from build123d import *

# Parameters (mm, degrees)
SKETCH_1_R                   = 12.5
EXTRUDE_1_DEPTH              = 20
HOLE_WIZARD_M2_1_D           = 2.4
HOLE_WIZARD_M2_1_CBORE_D     = 6
HOLE_WIZARD_M2_1_CBORE_DEPTH = 0.5


with BuildPart() as part:
    # 草图1 → 凸台-拉伸1 (new body)
    with BuildSketch(Plane.XY):
        Polygon((-340.66541114, -145.626712598), (-330.66541114, -145.626712598), (-330.66541114, -165), (-290.66541114, -165), (-290.66541114, -145.626712598), (-280.66541114, -145.626712598), (-280.66541114, -130), (-340.66541114, -130), align=None)
        with Locations((-310.66541114, -150)):
            Circle(SKETCH_1_R, mode=Mode.SUBTRACT)
    extrude(amount=EXTRUDE_1_DEPTH)

    # M2 六角头螺栓的柱形沉头孔1 (through all)
    with Locations(Plane(origin=(0, -145.626712598, 0), x_dir=(-1, 0, 0), z_dir=(0, -1, 0))):
        with Locations((335.897321014, -10), (285.620390856, -10)):
            CounterBoreHole(HOLE_WIZARD_M2_1_D / 2, HOLE_WIZARD_M2_1_CBORE_D / 2, HOLE_WIZARD_M2_1_CBORE_DEPTH)


solid = part.part
For this review, take the finished solid that the model builds, in its own axes (mm). A direction names the side the tool comes from. Give positions to 0.01 mm unless a question says otherwise; leave off trailing zeros. Loops run counter-clockwise (first coordinate to the right, second up) from the corner with the lowest first, then second, coordinate; pieces in that order, holes last. Notation, with made-up numbers: M 34,75.25 L 51,75.25 A28 cw 51,109.25 Z; hole C -31,-1 d10. An arc over 180 degrees is marked long. Answer as a JSON object with one key per item and string values. Group by question number.
Q1. Mouldability with a two-part tool opening along X and no side actions: class faces 1 (the flat face through (-280.665, -138, 10)), 2 (the flat face through (-311, -136, 20)), 3 (the flat face through (-337, -145.127, 11)), 4 (the flat face through (-287, -145.127, 10)) as +X half, -X half, draft (parallel to the pull), parting line (faces both ways), or undercut.
Q2. Add section A-A on z = 10. Give the boundary of the cut face in (x, y).
Q3. Add section C-C on z = 1.5. Give the boundary of the cut face in (x, y).
Q4. Add section B-B on y = -150. Give the boundary of the cut face in (x, z).
Q5. Tool access review of faces 5 (the flat face through (-333.5, -145.627, 7.6)), 6 (the cylindrical face through (-282.623, -145.38, 9.868)), 7 (the flat face through (-288, -145.627, 7.6)): name each direction out of +Z, -Z, +X, -X, +Y, -Y from which nothing blocks a thin tool from reaching the whole face with its end or side.
Q6. Insertion check: P1, Ø5, axis at x = -337, z = 13.5, coming from the -Y side; P2, Ø9.5, axis at y = -156.5, z = 10.5, coming from the -X side; P3, Ø3, axis at y = -151, z = 8, coming from the +X side; P4, Ø6, axis at x = -304.5, y = -155, coming from the -Z side. Each pin has a flat end and moves straight along its axis. Give the tip position at first contact, or say it passes through.
Q7. Add section D-D on x = -322. Give the boundary of the cut face in (y, z).
Q8. For probe 1 along X at (y, z) = (-136.5, 10); probe 2 along X at (y, z) = (-145.45, 10); probe 3 along X at (y, z) = (-141, 10), list the stretches that pass through material, from the lowest coordinate up. Write a range as [from, to].
Checked values:
{
 "1": {"face 1": "+X half", "face 2": "draft", "face 3": "undercut", "face 4": "undercut"},
 "2": {"outline": "M -340.67,-145.63 L -338.9,-145.63 L -338.9,-145.13 L -337.1,-145.13 L -337.1,-130 L -340.67,-130 Z; M -334.7,-145.13 L -332.9,-145.13 L -332.9,-145.63 L -330.67,-145.63 L -330.67,-165 L -290.67,-165 L -290.67,-145.63 L -288.62,-145.63 L -288.62,-145.13 L -286.82,-145.13 L -286.82,-130 L -334.7,-130 Z; M -284.42,-145.13 L -282.62,-145.13 L -282.62,-145.63 L -280.67,-145.63 L -280.67,-130 L -284.42,-130 Z; hole C -310.67,-150 d25"},
 "3": {"outline": "M -340.67,-145.63 L -330.67,-145.63 L -330.67,-165 L -290.67,-165 L -290.67,-145.63 L -280.67,-145.63 L -280.67,-130 L -340.67,-130 Z; hole C -310.67,-150 d25"},
 "4": {"outline": "M -330.67,0 L -323.17,0 L -323.17,20 L -330.67,20 Z; M -298.17,0 L -290.67,0 L -290.67,20 L -298.17,20 Z"},
 "5": {"face 5": "+Z, -Z, -X, -Y", "face 6": "-Y", "face 7": "+Z, -Z, +X, -Y"},
 "6": {"P1": "y = -145.63", "P2": "x = -330.67", "P3": "x = -290.67", "P4": "through"},
 "7": {"outline": "M -165,0 L -155.27,0 L -155.27,20 L -165,20 Z; M -144.73,0 L -130,0 L -130,20 L -144.73,20 Z"},
 "8": {"probe 1": "[-340.67, -337.1], [-334.7, -286.82], [-284.42, -280.67]", "probe 2": "[-340.67, -338.9], [-332.9, -322.31], [-299.02, -288.62], [-282.62, -280.67]", "probe 3": "[-340.67, -337.1], [-334.7, -319.34], [-301.99, -286.82], [-284.42, -280.67]"}
}
